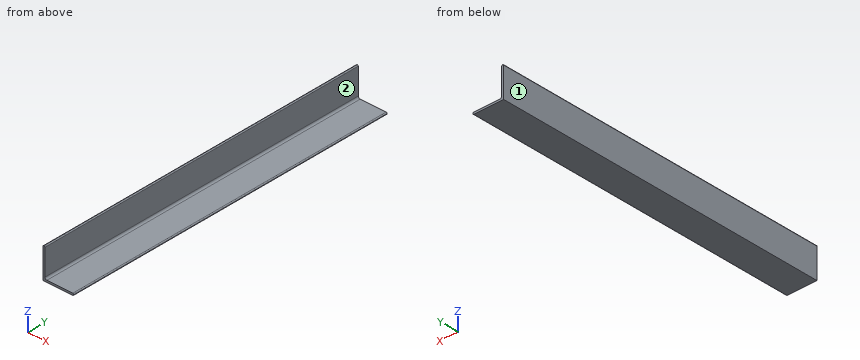
```python
from build123d import *

# Parameters (mm, degrees)
F1_DEPTH = 558.8


with BuildPart() as f1:
    # F0 (on Front) → F1 (new body)
    with BuildSketch(Plane.XZ):
        with BuildLine():
            Line((0, 49.276), (0, 0))
            Line((0, 0), (49.276, 0))
            ThreePointArc((49.276, 0), (50.353631, 0.446369), (50.8, 1.524))
            Line((50.8, 1.524), (50.8, 1.651))
            ThreePointArc((50.8, 1.651), (50.353631, 2.728631), (49.276, 3.175))
            Line((49.276, 3.175), (6.35, 3.175))
            ThreePointArc((6.35, 3.175), (4.104936, 4.104936), (3.175, 6.35))
            Line((3.175, 6.35), (3.175, 49.276))
            ThreePointArc((3.175, 49.276), (2.728631, 50.353631), (1.651, 50.8))
            Line((1.651, 50.8), (1.524, 50.8))
            ThreePointArc((1.524, 50.8), (0.446369, 50.353631), (0, 49.276))
        make_face()
    extrude(amount=F1_DEPTH)


solid = f1.part
```
Could you check a few things on this model? Use its own coordinates, in mm. Face numbers are marked on the shaded views. A direction names the side the tool comes from. Coordinates: 2 decimals unless noted, no trailing zeros. Write each loop counter-clockwise with the first axis right and the second up, starting at its lowest first coordinate (ties: lowest second). Pieces come first, ordered by that corner, then holes. Notation, with made-up numbers: M 9.25,48 L 45.25,48 A24 ccw 45.25,69 Z; hole C 12,-30 d11. An arc over 180 degrees is marked long. Answer as CSV lines item,"result". Start each with the question number.
1) For P1, Ø4, axis at x = 38.5, y = -452.5, coming from the +Z side (3 decimals); P2, Ø6, axis at y = -332.5, z = 40.5, coming from the +X side (3 decimals), each with a flat end and sliding along its axis, tell me the tip position at first contact or that it passes through.
2) I want a section at C-C, the plane z = 39. Please give me the cut outline in (x, y) (3 decimals), and give its area (3 significant figures).
3) I want a section at A-A, the plane y = -385. Please give me the cut outline in (x, z) (3 decimals).
4) Please list where these lines run through material, in increasing order: line 1 (Z direction, x = 7.5, y = -100) (3 decimals); line 2 (Z direction, x = 2, y = -309.5). Write a range as from..to.
5) For the marked faces 1 and 2, which set-ups out of +Z, -Z, +X, -X, +Y, -Y let a thin tool reach every point of the face, with its end or its side?
6) I want a section at B-B, the plane x = 25. Please give me the cut outline in (y, z) (3 decimals).
Data:
1,P1,"stops at z = 3.175"
1,P2,"stops at x = 3.175"
2,outline,"M 0,-558.8 L 3.175,-558.8 L 3.175,0 L 0,0 Z"
2,area,"1,770 mm^2"
3,outline,"M 0,0 L 49.276,0 A1.524 ccw 50.8,1.524 L 50.8,1.651 A1.524 ccw 49.276,3.175 L 6.35,3.175 A3.175 cw 3.175,6.35 L 3.175,49.276 A1.524 ccw 1.651,50.8 L 1.524,50.8 A1.524 ccw 0,49.276 Z"
4,line 1,"z = 0..3.175"
4,line 2,"z = 0..50.76"
5,face 1,"+Z, -Z, -X, +Y, -Y"
5,face 2,"+Z, +X, +Y, -Y"
6,outline,"M -558.8,0 L 0,0 L 0,3.175 L -558.8,3.175 Z"
